```python
from build123d import *

# Parameters (mm, degrees)
F0_W     = 106
F0_H     = 37
F0_R     = 13.5
F1_DEPTH = 10
F2_DEPTH = 3


with BuildPart() as f1:
    # F0 (on Top) → F1 (new body)
    with BuildSketch(Plane.XY):
        Rectangle(F0_W, F0_H)
        with Locations((-34.5, 0)):
            Circle(F0_R, mode=Mode.SUBTRACT)
        Circle(F0_R, mode=Mode.SUBTRACT)
        with Locations((34.5, 0)):
            Circle(F0_R, mode=Mode.SUBTRACT)
    extrude(amount=F1_DEPTH)

    # F0 (on Top) → F2 (join)
    with BuildSketch(Plane.XY):
        Circle(F0_R)
        with Locations((-34.5, 0)):
            Circle(F0_R)
        with Locations((34.5, 0)):
            Circle(F0_R)
    extrude(amount=F2_DEPTH)


solid = f1.part
```
Build history of the part. All positions in model axes, mm. A direction names the side the tool comes from. Give positions to 0.01 mm unless a question says otherwise; leave off trailing zeros. Loops run counter-clockwise (first coordinate to the right, second up) from the corner with the lowest first, then second, coordinate; pieces in that order, holes last.
1) 3-axis set-ups, long thin cutter, end or side, ignore diameter. For faces 4 (the face through (-13, 8, 10)), 5 (the face through (-35, 0, 3)): which of +Z, -Z, +X, -X, +Y, -Y reach the whole face in a straight line?
Values follow:
face 4: +Z, +X, -X, +Y, -Y
face 5: +Z
2) Drop a flat-ended pin along its axis: P1, Ø8, axis at x = 6.5, y = 6, coming from the +Z side. Give the stop position or say it passes through.
Values follow:
P1: stops at z = 3
3) Band-saw the part on A-A on x = -34.5. List the corners of the cut face in (y, z), then the cut area to 3 significant figures.
Values follow:
outline: (-18.5, 0) - (18.5, 0) - (18.5, 10) - (13.5, 10) - (13.5, 3) - (-13.5, 3) - (-13.5, 10) - (-18.5, 10) - close
area: 181 mm2
4) Band-saw the part on C-C on y = 0. List the corners of the cut face in (x, z).
Values follow:
outline: (-53, 0) - (53, 0) - (53, 10) - (48, 10) - (48, 3) - (21, 3) - (21, 10) - (13.5, 10) - (13.5, 3) - (-13.5, 3) - (-13.5, 10) - (-21, 10) - (-21, 3) - (-48, 3) - (-48, 10) - (-53, 10) - close
5) Band-saw the part on D-D on x = 12.5. List the corners of the cut face in (y, z).
Values follow:
outline: (-18.5, 0) - (18.5, 0) - (18.5, 10) - (5.1, 10) - (5.1, 3) - (-5.1, 3) - (-5.1, 10) - (-18.5, 10) - close
6) Band-saw the part on B-B on z = 7.25. List the corners of the cut face in (x, y), then the cut area to 3 significant figures.
Values follow:
outline: (-53, -18.5) - (53, -18.5) - (53, 18.5) - (-53, 18.5) - close; hole circle Ø27 at (-34.5, 0); hole circle Ø27 at (0, 0); hole circle Ø27 at (34.5, 0)
area: 2,200 mm2
7) Two-plate mould, pull along Y, no slides. Class faces 1 (the face through (-1, -18.5, 5)), 2 (the face through (53, 0, 5)), 3 (the face through (0, 0, 3)): released by +Y, released by -Y, zero draft, split by the parting line, or undercut.
Values follow:
face 1: released by -Y
face 2: zero draft
face 3: undercut
8) Probe line 1 along Y through (x, z) = (34.5, 6.25); line 2 along X through (y, z) = (-11.5, 7.5); line 3 along X through (y, z) = (9, 7). List the from-to ranges inside material, lowest first.
Values follow:
line 1: y = -18.5 to -13.5, 13.5 to 18.5
line 2: x = -53 to -41.57, -27.43 to -7.07, 7.07 to 27.43, 41.57 to 53
line 3: x = -53 to -44.56, -24.44 to -10.06, 10.06 to 24.44, 44.56 to 53
